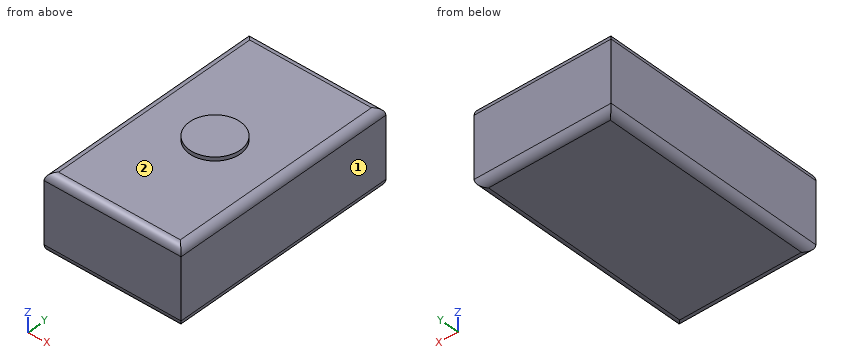
```python
from build123d import *

# Parameters (mm, degrees)
F0_W     = 457.2
F0_H     = 762
F1_DEPTH = 254
F2_R     = 25.4
F3_R     = 84.662074
F4_DEPTH = 12.7


with BuildPart() as f1:
    # F0 (on Top) → F1 (new body)
    with BuildSketch(Plane.XY):
        Rectangle(F0_W, F0_H)
    extrude(amount=F1_DEPTH)

    # F2
    f2_edges = [f1.edges().sort_by_distance(p)[0] for p in [
        (0, 381, 254),
        (228.6, 0, 254),
        (0, -381, 254),
        (-228.6, 0, 254),
        (228.6, 0, 0),
        (-228.6, 0, 0),
        (0, -381, 0),
        (0, 381, 0),
    ]]
    fillet(f2_edges, radius=F2_R)

    # F3 (on face) → F4 (join)
    with BuildSketch(Plane.XY.offset(254)):
        Circle(F3_R)
    extrude(amount=F4_DEPTH)


solid = f1.part
```
The listing builds one solid part. Answer for the finished solid, in the listing's coordinates (mm). Face numbers are marked on the shaded views. A direction names the side the tool comes from. Coordinates: 2 decimals unless noted, no trailing zeros. Loops run counter-clockwise (first coordinate to the right, second up) from the corner with the lowest first, then second, coordinate; pieces in that order, holes last. Notation, with made-up numbers: M 65,-11 L 73,-11 A27 cw 73,18 Z; hole C 77,-24 d7. An arc over 180 degrees is marked long. Answer as a JSON object with one key per item and string values. Group by question number.
Item 1: Which of the six approach directions +Z, -Z, +X, -X, +Y, -Y give full straight-line access (tool end or side, diameter ignored) to the marked faces 1 and 2?
Item 2: Section A-A (y = 201) is taken. Write down the section's boundary in (x, z).
Item 3: Section C-C (y = 0) is taken. Write down the section's boundary in (x, z).
Item 4: Section D-D (x = -172) is taken. Write down the section's boundary in (y, z).
Item 5: Section B-B (x = 0) is taken. Write down the section's boundary in (y, z).
Item 6: This flat-tipped pin is pushed along its axis until it touches: P1, Ø8, axis at x = -91.5, y = -265, coming from the +Z side. Where does it stop, or does it pass through?
Item 7: Consider L1, parallel to Y at x = 171, z = 23; L2, parallel to Z at x = -111, y = -61; L3, parallel to Y at x = 12, z = 229.5. Determine where each line is inside the solid, lowest interval first.
Solved:
{
 "1": {"face 1": "+Z, -Z, +X, +Y, -Y", "face 2": "+Z"},
 "2": {"outline": "M -228.6,25.4 A25.4 ccw -203.2,0 L 203.2,0 A25.4 ccw 228.6,25.4 L 228.6,228.6 A25.4 ccw 203.2,254 L -203.2,254 A25.4 ccw -228.6,228.6 Z"},
 "3": {"outline": "M -228.6,25.4 A25.4 ccw -203.2,0 L 203.2,0 A25.4 ccw 228.6,25.4 L 228.6,228.6 A25.4 ccw 203.2,254 L 84.66,254 L 84.66,266.7 L -84.66,266.7 L -84.66,254 L -203.2,254 A25.4 ccw -228.6,228.6 Z"},
 "4": {"outline": "M -381,25.4 A25.4 ccw -355.6,0 L 355.6,0 A25.4 ccw 381,25.4 L 381,228.6 A25.4 ccw 355.6,254 L -355.6,254 A25.4 ccw -381,228.6 Z"},
 "5": {"outline": "M -381,25.4 A25.4 ccw -355.6,0 L 355.6,0 A25.4 ccw 381,25.4 L 381,228.6 A25.4 ccw 355.6,254 L 84.66,254 L 84.66,266.7 L -84.66,266.7 L -84.66,254 L -355.6,254 A25.4 ccw -381,228.6 Z"},
 "6": {"P1": "stops at z = 254"},
 "7": {"L1": "y = -380.89 to 380.89", "L2": "z = 0 to 254", "L3": "y = -380.98 to 380.98"}
}
